Geometry: final body of the model. Coordinates: model frame, mm. Coordinates: 2 decimals unless noted, no trailing zeros. Write each loop counter-clockwise with the first axis right and the second up, starting at its lowest first coordinate (ties: lowest second). Pieces come first, ordered by that corner, then holes. Notation, with made-up numbers: (-25.5, 58) - (20.5, 58) arc R25 ccw to (20.5, 73) - close; hole circle Ø8 at (35, 31). An arc over 180 degrees is marked (long way). Answer as a JSON object with one key per item and string values. Group by question number.
Item 1: Section B-B on x = 30.5. Return loops of the section in (y, z), and give its area (3 significant figures).
Item 2: First-contact query: pin 1 Ø1.2 at (x, z) = (-49.5, 1.5) entering from +Y; pin 2 Ø2 at (y, z) = (-49, 1.5) entering from +X; pin 3 Ø2 at (x, z) = (33.5, 1.5) entering from -Y. Flat tips, straight axial feed; report the tip coordinate or a pass-through.
Item 3: Line query: line 1 along X through (y, z) = (-28, 0.35); line 2 along Y through (x, z) = (-50, 2.15). Output: solid intervals per line, ascending. Write a range as from..to.
Item 4: Section A-A on y = -24.5. Return loops of the section in (x, z).
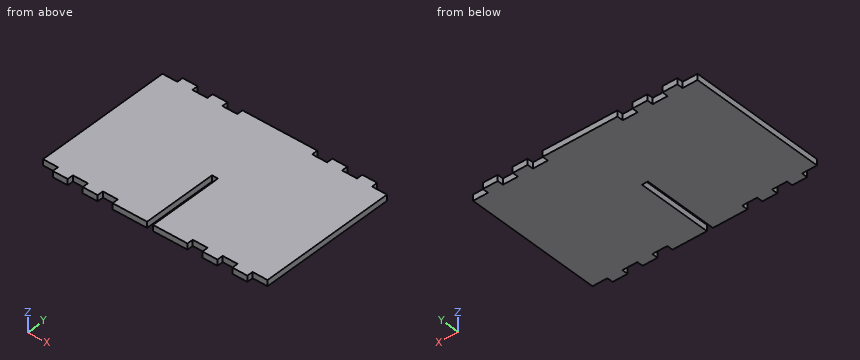
```python
from build123d import *

# Parameters (mm, degrees)
SKETCH1_W           = 150
SKETCH1_H           = 100
BOSS_EXTRUDE1_DEPTH = 4
CUT_EXTRUDE2_START  = 4
SKETCH3_W           = 10
SKETCH3_H           = 4
SKETCH3_W_2         = 4
SKETCH3_H_2         = 50
CUT_EXTRUDE2_DEPTH  = 5


with BuildPart() as part:
    # Sketch1 → Boss-Extrude1 (new body)
    with BuildSketch(Plane.XY):
        Rectangle(SKETCH1_W, SKETCH1_H)
    extrude(amount=BOSS_EXTRUDE1_DEPTH)

    # Sketch3 → Cut-Extrude2 (cut, through all)
    with BuildSketch(Plane.XY.offset(CUT_EXTRUDE2_START)):
        with Locations((-50, 48)):
            Rectangle(SKETCH3_W, SKETCH3_H)
        with Locations((-30, 48)):
            Rectangle(SKETCH3_W, SKETCH3_H)
        with Locations((-70, 48)):
            Rectangle(SKETCH3_W, SKETCH3_H)
        with Locations((70, 48)):
            Rectangle(SKETCH3_W, SKETCH3_H)
        with Locations((50, 48)):
            Rectangle(SKETCH3_W, SKETCH3_H)
        with Locations((30, 48)):
            Rectangle(SKETCH3_W, SKETCH3_H)
        with Locations((50, -48)):
            Rectangle(SKETCH3_W, SKETCH3_H)
        with Locations((30, -48)):
            Rectangle(SKETCH3_W, SKETCH3_H)
        with Locations((70, -48)):
            Rectangle(SKETCH3_W, SKETCH3_H)
        with Locations((-70, -48)):
            Rectangle(SKETCH3_W, SKETCH3_H)
        with Locations((-50, -48)):
            Rectangle(SKETCH3_W, SKETCH3_H)
        with Locations((-30, -48)):
            Rectangle(SKETCH3_W, SKETCH3_H)
        with Locations((0, -25)):
            Rectangle(SKETCH3_W_2, SKETCH3_H_2)
    extrude(amount=-CUT_EXTRUDE2_DEPTH, mode=Mode.SUBTRACT)


solid = part.part
```
Checks:
{
 "1": {"outline": "(-46, 0) - (46, 0) - (46, 4) - (-46, 4) - close", "area": "368 mm^2"},
 "2": {"pin 1": "y = 46", "pin 2": "x = 65", "pin 3": "y = -46"},
 "3": {"line 1": "-75..-2, 2..75", "line 2": "-46..46"},
 "4": {"outline": "(-75, 0) - (-2, 0) - (-2, 4) - (-75, 4) - close; (2, 0) - (75, 0) - (75, 4) - (2, 4) - close"}
}
